Could you check a few things on this model? Use its own coordinates, in mm. A direction names the side the tool comes from. Give positions to 0.01 mm unless a question says otherwise; leave off trailing zeros. Write each loop counter-clockwise with the first axis right and the second up, starting at its lowest first coordinate (ties: lowest second). Pieces come first, ordered by that corner, then holes. Notation, with made-up numbers: M -14.75,5.25 L 29.25,5.25 A33 cw 29.25,38.25 Z; hole C 38,44.25 d11. An arc over 180 degrees is marked long. Use one line per item in the form item = value.
from build123d import *

# Parameters (mm, degrees)
SKETCH1_W                  = 80.3
SKETCH1_H                  = 66
BOSS_EXTRUDE1_DEPTH        = 3
FILLET1_R                  = 3.5
SKETCH2_R                  = 3.5
CUT_EXTRUDE1_DEPTH         = 4
FILLET2_R                  = 3.5
F_3_5_3_5_DIAMETER_HOLE1_D = 3.5


with BuildPart() as part:
    # Sketch1 → Boss-Extrude1 (new body)
    with BuildSketch(Plane.XY):
        Polygon((-18, -20), (60.3, -20), (80.3, 0), (0, 0), (0, 66), (-18, 48), align=None)
        with Locations((40.15, 33)):
            Rectangle(SKETCH1_W, SKETCH1_H)
    extrude(amount=BOSS_EXTRUDE1_DEPTH)

    # Fillet1
    fillet1_edges = [part.edges().sort_by_distance(p)[0] for p in [
        (60.3, -20, 1.5),
        (-18, -20, 1.5),
        (-18, 48, 1.5),
        (0, 66, 1.5),
        (80.3, 66, 1.5),
        (80.3, 0, 1.5),
    ]]
    fillet(fillet1_edges, radius=FILLET1_R)

    # Sketch2 → Cut-Extrude1 (cut, through all)
    with BuildSketch(Plane.XY.offset(3)):
        with BuildLine():
            Line((0, 62.5), (0, 0))
            Line((0, 0), (76.8, 0))
            ThreePointArc((76.8, 0), (74.325126266, 5.974873734), (80.3, 3.5))
            Line((80.3, 3.5), (80.3, 62.5))
            ThreePointArc((80.3, 62.5), (74.325126266, 60.025126266), (76.8, 66))
            Line((76.8, 66), (3.500000005, 66))
            ThreePointArc((3.500000005, 66), (5.974873736, 64.974873732), (7, 62.5))
            ThreePointArc((7, 62.5), (3.5, 59), (0, 62.5))
        make_face()
        with Locations((3.5, 62.5)):
            Circle(SKETCH2_R)
        with BuildLine():
            ThreePointArc((76.8, 66), (74.325126266, 60.025126266), (80.3, 62.5))
            ThreePointArc((80.3, 62.5), (79.274873734, 64.974873734), (76.8, 66))
        make_face()
        with Locations((76.8, 3.5)):
            Circle(SKETCH2_R)
    extrude(amount=-CUT_EXTRUDE1_DEPTH, mode=Mode.SUBTRACT)

    # Fillet2
    fillet2_edges = [part.edges().sort_by_distance(p)[0] for p in [
        (0, 0, 1.5),
    ]]
    fillet(fillet2_edges, radius=FILLET2_R)

    # Ø3.5 (3.5) Diameter Hole1 (through all)
    with Locations(Plane.XY.offset(3)):
        with Locations((67.24, -4.57)):
            Hole(F_3_5_3_5_DIAMETER_HOLE1_D / 2)


solid = part.part
1) I want a section at B-B, the plane z = 2.1. Please give me the cut outline in (x, y).
Checked values:
outline = M -18,-16.5 A3.5 ccw -14.5,-20 L 58.85,-20 A3.5 ccw 61.33,-18.97 L 79.27,-1.03 A3.5 ccw 80.3,1.45 L 80.3,3.5 A3.5 cw 76.8,0 L 3.5,0 A3.5 cw 0,3.5 L 0,62.5 A3.5 cw 3.5,66 L 1.45,66 A3.5 ccw -1.03,64.97 L -16.97,49.03 A3.5 ccw -18,46.55 Z; hole C 67.24,-4.57 d3.5
2) If I drill on L1, parallel to X at y = 37, z = 2; L2, parallel to Y at x = 19, z = 1.1; L3, parallel to Y at x = 67.24, z = 2, over which ranges is the centre line in solid material (lowest first)?
Checked values:
L1 = -18 to 0
L2 = -20 to 0
L3 = -13.06 to -6.32, -2.82 to 0
3) For faces 5 (the flat face through (0, 33, 2)), 6 (the flat face through (-9, 57, 1)), 7 (the flat face through (80.3, 2, 1)), 8 (the flat face through (40, 0, 2)), 9 (the cylindrical face through (1, 1.05, 1.48)), which set-ups out of +Z, -Z, +X, -X, +Y, -Y let a thin tool reach every point of the face, with its end or its side?
Checked values:
face_5 = +Z, -Z, +X
face_6 = +Z, -Z, -X, +Y
face_7 = +Z, -Z, +X, +Y, -Y
face_8 = +Z, -Z, +Y
face_9 = +Z, -Z
4) I want a section at A-A, the plane y = -4.57. Please give me the cut outline in (x, z).
Checked values:
outline = M -18,0 L 65.49,0 L 65.49,3 L -18,3 Z; M 68.99,0 L 75.73,0 L 75.73,3 L 68.99,3 Z
5) Thinking about a two-plate mould opening in X: for faces 1 (the flat face through (9, -5, 0)), 2 (the flat face through (70.2, -10.1, 1.5)), 3 (the cylindrical face through (79.25, 1, 1.52)), 4 (the cylindrical face through (68.99, -4.49, 1.48)), which applies, released by +X, released by -X, zero draft, split by the parting line, or undercut?
Checked values:
face_1 = zero draft
face_2 = released by +X
face_3 = undercut
face_4 = undercut
6) For pin 1 Ø3 at (x, y) = (67.24, -4.57) entering from -Z; pin 2 Ø1 at (x, z) = (43.5, 1) entering from +Y; pin 3 Ø1.5 at (y, z) = (30, 1) entering from +X, each with a flat end and sliding along its axis, tell me the tip position at first contact or that it passes through.
Checked values:
pin_1 = through
pin_2 = 0
pin_3 = 0
7) I want a section at D-D, the plane x = 7. Please give me the cut outline in (y, z), plus the area to 3 significant figures.
Checked values:
outline = M -20,0 L 0,0 L 0,3 L -20,3 Z
area = 60.0 mm2
8) I want a section at C-C, the plane x = 67.24. Please give me the cut outline in (y, z).
Checked values:
outline = M -13.06,0 L -6.32,0 L -6.32,3 L -13.06,3 Z; M -2.82,0 L 0,0 L 0,3 L -2.82,3 Z
